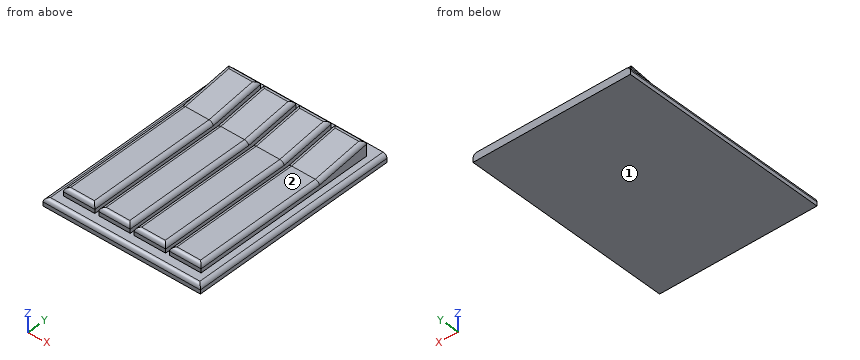
from build123d import *

# Parameters (mm, degrees)
F0_W         = 10.16
F0_H         = 17.20733324
F1_DEPTH     = 7.62
F0_H_2       = 42.8125401959
F2_DEPTH     = 5.08
F0_W_2       = 50.8
F0_H_3       = 67.63987211
F3_DEPTH     = 2.54
F4_T4_DEPTH  = 102.5816286105
F4_T9_DEPTH  = 102.5816286105
F4_T14_DEPTH = 102.5816286105
F4_T19_DEPTH = 102.5816286105
F5_R         = 1.27
F6_R         = 1.27


# Not quite as in the source:
# - a fillet or chamfer that OpenCascade refuses, or shapes differently, is made with other operations: its cross-section is extruded or revolved along the edge and cut away or added
# - two fillets or chamfers of one size are made in one step
# - ends of sketch curves that miss each other by under 0.0002 mm in the source are joined


with BuildPart() as f1:
    # F0 (on Top) → F1 (new body)
    with BuildSketch(Plane.XY):
        with Locations((-17.1449951105, 21.4062702746)):
            Rectangle(F0_W, F0_H)
    extrude(amount=F1_DEPTH)

    # F0 (on Top) → F2 (join)
    with BuildSketch(Plane.XY):
        with Locations((-17.1449951105, 21.4062702746)):
            Rectangle(F0_W, F0_H)
        with Locations((-17.1449951105, -8.6036664434)):
            Rectangle(F0_W, F0_H_2)
    extrude(amount=F2_DEPTH)



with BuildPart() as f1b:
    # F0 (on Top) → F1, piece 2 (new body)
    with BuildSketch(Plane.XY):
        with Locations((-5.7149951105, 21.4062702746)):
            Rectangle(F0_W, F0_H)
    extrude(amount=F1_DEPTH)

    # F0 (on Top) → F2, piece 2 (join)
    with BuildSketch(Plane.XY):
        with Locations((-5.7149951105, -8.6036664434)):
            Rectangle(F0_W, F0_H_2)
        with Locations((-5.7149951105, 21.4062702746)):
            Rectangle(F0_W, F0_H)
    extrude(amount=F2_DEPTH)


with BuildPart() as f1c:
    # F0 (on Top) → F1, piece 3 (new body)
    with BuildSketch(Plane.XY):
        with Locations((5.7150048895, 21.4062702746)):
            Rectangle(F0_W, F0_H)
    extrude(amount=F1_DEPTH)

    # F0 (on Top) → F2, piece 3 (join)
    with BuildSketch(Plane.XY):
        with Locations((5.7150048895, -8.6036664434)):
            Rectangle(F0_W, F0_H_2)
        with Locations((5.7150048895, 21.4062702746)):
            Rectangle(F0_W, F0_H)
    extrude(amount=F2_DEPTH)


with BuildPart() as f1d:
    # F0 (on Top) → F1, piece 4 (new body)
    with BuildSketch(Plane.XY):
        with Locations((17.1450048895, 21.4062702746)):
            Rectangle(F0_W, F0_H)
    extrude(amount=F1_DEPTH)

    # F0 (on Top) → F2, piece 4 (join)
    with BuildSketch(Plane.XY):
        with Locations((17.1450048895, -8.6036664434)):
            Rectangle(F0_W, F0_H_2)
        with Locations((17.1450048895, 21.4062702746)):
            Rectangle(F0_W, F0_H)
    extrude(amount=F2_DEPTH)


with BuildPart() as f1_1:
    add(f1.part)

    add(f1b.part)  # F3 merges F1b

    add(f1c.part)  # F3 merges F1c

    add(f1d.part)  # F3 merges F1d
    # F0 (on Top) → F3 (join)
    with BuildSketch(Plane.XY):
        with Locations((0, -1.609e-07)):
            Rectangle(F0_W_2, F0_H_3)
        Polygon((-22.2249951105, 30.0099368946), (-12.0649951105, 30.0099368946), (-12.0649951105, 12.8026036546), (-12.0649951105, -30.0099365413), (-22.2249951105, -30.0099365413), (-22.2249951105, 12.8026036546), align=None, mode=Mode.SUBTRACT)
        Polygon((-10.7949951105, -30.0099365413), (-10.7949951105, 12.8026036546), (-10.7949951105, 30.0099368946), (-0.6349951105, 30.0099368946), (-0.6349951105, 12.8026036546), (-0.6349951105, -30.0099365413), align=None, mode=Mode.SUBTRACT)
        Polygon((0.6350048895, -30.0099365413), (0.6350048895, 12.8026036546), (0.6350048895, 30.0099368946), (10.7950048895, 30.0099368946), (10.7950048895, 12.8026036546), (10.7950048895, -30.0099365413), align=None, mode=Mode.SUBTRACT)
        Polygon((12.0650048895, -30.0099365413), (12.0650048895, 12.8026036546), (12.0650048895, 30.0099368946), (22.2250048895, 30.0099368946), (22.2250048895, 12.8026036546), (22.2250048895, -30.0099365413), align=None, mode=Mode.SUBTRACT)
    extrude(amount=F3_DEPTH)

    # F4: chamfer of 17.78 x 2.54 on 4 edges, made by hand


with BuildPart() as f4_tool2:
    # F4_s3 → F4_t4 (new body)
    with BuildSketch(Plane.YZ.offset(-68.4358094158)):
        Polygon((30.5826036546, 7.62), (12.8026036546, 5.08), (12.8026036546, 7.62), align=None)
    extrude(amount=F4_T4_DEPTH)

    split(bisect_by=Plane.XY.offset(5.08), keep=Keep.TOP)


with BuildPart() as f1_2:
    add(f1_1.part)

    # F4_t1: cut F4_tool2
    add(f4_tool2.part, mode=Mode.SUBTRACT)


with BuildPart() as f4_tool7:
    # F4_s8 → F4_t9 (new body)
    with BuildSketch(Plane.YZ.offset(-57.0058094158)):
        Polygon((12.8026036546, 5.08), (30.5826036546, 7.62), (12.8026036546, 7.62), align=None)
    extrude(amount=F4_T9_DEPTH)

    split(bisect_by=Plane.XY.offset(5.08), keep=Keep.TOP)


with BuildPart() as f1_3:
    add(f1_2.part)

    # F4_t6: cut F4_tool7
    add(f4_tool7.part, mode=Mode.SUBTRACT)


with BuildPart() as f4_tool12:
    # F4_s13 → F4_t14 (new body)
    with BuildSketch(Plane.YZ.offset(-45.5758094158)):
        Polygon((12.8026036546, 5.08), (30.5826036546, 7.62), (12.8026036546, 7.62), align=None)
    extrude(amount=F4_T14_DEPTH)

    split(bisect_by=Plane.XY.offset(5.08), keep=Keep.TOP)


with BuildPart() as f1_4:
    add(f1_3.part)

    # F4_t11: cut F4_tool12
    add(f4_tool12.part, mode=Mode.SUBTRACT)


with BuildPart() as f4_tool17:
    # F4_s18 → F4_t19 (new body)
    with BuildSketch(Plane.YZ.offset(-34.1458094158)):
        Polygon((12.8026036546, 5.08), (30.5826036546, 7.62), (12.8026036546, 7.62), align=None)
    extrude(amount=F4_T19_DEPTH)

    split(bisect_by=Plane.XY.offset(5.08), keep=Keep.TOP)


with BuildPart() as f1_5:
    add(f1_4.part)

    # F4_t16: cut F4_tool17
    add(f4_tool17.part, mode=Mode.SUBTRACT)

    # F5
    f5_edges = [f1_5.edges().sort_by_distance(p)[0] for p in [
        (0, -33.819936, 2.54),
        (-25.4, 0, 2.54),
        (25.4, 0, 2.54),
    ]]
    fillet(f5_edges, radius=F5_R)

    # F6
    f6_edges = [f1_5.edges().sort_by_distance(p)[0] for p in [
        (-12.064995, -8.603666, 5.08),
        (-17.144995, -30.009937, 5.08),
        (-22.224995, -8.603666, 5.08),
        (-5.714995, -30.009937, 5.08),
        (-10.794995, -8.603666, 5.08),
        (-0.634995, -8.603666, 5.08),
        (0.635005, -8.603666, 5.08),
        (10.795005, -8.603666, 5.08),
        (5.715005, -30.009937, 5.08),
        (17.145005, -30.009937, 5.08),
        (12.065005, -8.603666, 5.08),
        (22.225005, -8.603666, 5.08),
        (-17.144995, 30.009937, 7.53819),
        (-12.064995, 21.40627, 6.309095),
        (-22.224995, 21.40627, 6.309095),
        (-10.794995, 21.40627, 6.309095),
        (-5.714995, 30.009937, 7.53819),
        (-0.634995, 21.40627, 6.309095),
        (0.635005, 21.40627, 6.309095),
        (5.715005, 30.009937, 7.53819),
        (10.795005, 21.40627, 6.309095),
        (12.065005, 21.40627, 6.309095),
        (17.145005, 30.009937, 7.53819),
        (22.225005, 21.40627, 6.309095),
    ]]
    fillet(f6_edges, radius=F6_R)


solid = f1_5.part
Work out the finished part from the listing and answer in its coordinate system (mm). Face numbers are marked on the shaded views. A direction names the side the tool comes from. Give positions to 0.01 mm unless a question says otherwise; leave off trailing zeros. Loops run counter-clockwise (first coordinate to the right, second up) from the corner with the lowest first, then second, coordinate; pieces in that order, holes last. Notation, with made-up numbers: (-39.75, 25) -> (-21.75, 25) arc R26 cw to (-21.75, 42) -> close; hole circle Ø9 at (2, 38). An arc over 180 degrees is marked (long way). Use a Markdown table: item, result. Add a question column.
1) The part is cut by section B-B, the plane x = 18. Determine the outline of the cut face in (y, z), plus the area to 3 significant figures.
2) Each of these flat-tipped pins is pushed along its axis until it touches: P1, Ø4, axis at y = 9.5, z = 4, coming from the +X side; P2, Ø24, axis at x = -11.5, y = 1.5, coming from the +Z side; P3, Ø4, axis at x = 17, y = -14.5, coming from the +Z side. Where does it stop, or does it pass through?
3) Which of the six approach directions +Z, -Z, +X, -X, +Y, -Y give full straight-line access (tool end or side, diameter ignored) to the marked faces 1 and 2?
4) Consider line 1 along X through (y, z) = (-5.5, 3) (3 decimals); line 2 along X through (y, z) = (-28, 4.25); line 3 along Z through (x, y) = (8.5, -8). Determine where each line is inside the solid, lowest interval first.
Reported:
| question | item | result |
|---|---|---|
| 1 | outline | (-33.82, 0) -> (33.82, 0) -> (33.82, 2.54) -> (30.01, 2.54) -> (30.01, 6.07) arc R1.27 ccw to (28.56, 7.33) -> (12.8, 5.08) -> (-28.74, 5.08) arc R1.27 ccw to (-30.01, 3.81) -> (-30.01, 2.54) -> (-32.55, 2.54) arc R1.27 ccw to (-33.82, 1.27) -> close |
| 1 | area | 344 mm^2 |
| 2 | P1 | stops at x = 25.17 |
| 2 | P2 | stops at z = 5.16 |
| 2 | P3 | stops at z = 5.08 |
| 3 | face 1 | -Z, +X, -X, +Y, -Y |
| 3 | face 2 | +Z, +X, -X, -Y |
| 4 | line 1 | x = -22.225 to -12.065, -10.795 to -0.635, 0.635 to 10.795, 12.065 to 22.225 |
| 4 | line 2 | x = -22.15 to -12.14, -10.72 to -0.71, 0.71 to 10.72, 12.14 to 22.15 |
| 4 | line 3 | z = 0 to 5.08 |
